Autodesk Fusion 360 part; units mm, degrees
sketch "Sketch1" plane through (0, 0, 0) normal (0, 0, 1) x (1, 0, 0)
  line L0 (-27.1259, 29.8327) -> (51.8741, 29.8327)
  line L1 (51.8741, 29.8327) -> (51.8741, -62.1673)
  line L2 (51.8741, -62.1673) -> (-27.1259, -62.1673)
  line L3 (-27.1259, -62.1673) -> (-27.1259, 29.8327)
  line L4 (62.3741, -72.1673) -> (-36.6259, -72.1673)
  line L5 (-36.6259, -72.1673) -> (-36.6259, 39.8327)
  line L6 (-36.6259, 39.8327) -> (62.3741, 39.8327)
  line L7 (62.3741, 39.8327) -> (62.3741, -72.1673)
  line L8 (62.3741, -72.1673) -> (-36.6259, 39.8327) construction
  line L9 (-36.6259, -72.1673) -> (62.3741, 39.8327) construction
  circle A0 centre (-31.6259, -67.1673) radius 1.7
  circle A1 centre (-31.6259, 34.8327) radius 1.7
  circle A2 centre (57.3741, 34.8327) radius 1.7
  circle A3 centre (57.3741, -67.1673) radius 1.7
  circle A4 centre (-31.6259, 34.8327) radius 3
  circle A5 centre (57.3741, 34.8327) radius 3
  circle A6 centre (57.3741, -67.1673) radius 3
  circle A7 centre (-31.6259, -67.1673) radius 3
  point P0 (12.8741, -16.1673)
  dimension "d1" = 79
  dimension "d3" = 99
  dimension "d4" = 112
  dimension "d13" = 3.4
  dimension "d14" = 5
  dimension "d15" = 5
  dimension "d16" = 9.5
  dimension "d17" = 6
  dimension "d18" = 6
  dimension "d19" = 6
  dimension "d20" = 6
extrude "Extrude1" add sketch "Sketch1" along normal blind 9.9 from surface at 3.1 contours A4 | A5 | A6 | A7 makes body 1 at (-34.6222, 34.6832, 9.7) makes body 2 at (-34.3904, -68.3326, 9.7) makes body 3 at (54.3778, 34.6832, 9.7) makes body 4 at (54.8142, -68.7316, 9.7)
extrude "Extrude2" add sketch "Sketch1" along normal blind 13 contours L4 L5 L6 L7 bodies 1 2 3 4
extrude "Extrude3" add sketch "Sketch1" along normal blind 3 contours L0 L1 L2 L3 bodies 1
sketch "Sketch2" plane through (0, 0, 13) normal (0, 0, 1) x (-1, 0, 0)
  circle A0 centre (31.6259, -34.8327) radius 1.7
  circle A1 centre (-57.3741, 67.1673) radius 1.7
  line L0 (-51.8741, 62.1673) -> (27.1259, 62.1673)
  line L1 (27.1259, 62.1673) -> (27.1259, -29.8327)
  line L2 (27.1259, -29.8327) -> (-51.8741, -29.8327)
  line L3 (-51.8741, -29.8327) -> (-51.8741, 62.1673)
  line L4 (-62.3741, -39.8327) -> (36.6259, -39.8327)
  line L5 (36.6259, -39.8327) -> (36.6259, 72.1673)
  line L6 (36.6259, 72.1673) -> (-62.3741, 72.1673)
  line L7 (-62.3741, 72.1673) -> (-62.3741, -39.8327)
  circle A2 centre (31.6259, 67.1673) radius 1.7
  circle A3 centre (-57.3741, -34.8327) radius 1.7
  line L8 (-3.6241, 62.1673) -> (-22.1241, 62.1673)
  line L9 (-22.1241, 62.1673) -> (-22.1241, 72.1673)
  line L10 (-22.1241, 72.1673) -> (-3.6241, 72.1673)
  line L11 (-3.6241, 72.1673) -> (-3.6241, 62.1673)
  line L12 (-3.6241, 62.1673) -> (-22.1241, 72.1673) construction
  line L13 (-22.1241, 62.1673) -> (-3.6241, 72.1673) construction
  point P0 (-12.8741, 67.1673)
  dimension "d28" = 18.5
extrude "Extrude4" cut sketch "Sketch2" against normal blind 7.5 contours L0 L6 L8 L9 L10 L11 bodies 1
fillet "Fillet1" radius 5 1 edges at (-36.6259, 39.8327, 6.5) on bodies 1
fillet "Fillet2" radius 5 3 edges at (62.3741, 39.8327, 6.5) (62.3741, -72.1673, 6.5) (-36.6259, -72.1673, 6.5) on bodies 1
Model file for the job. Use its own axes, mm. A direction names the side the tool comes from. Round coordinates to 2 decimals unless told otherwise and drop trailing zeros. Loops run counter-clockwise (first coordinate to the right, second up) from the corner with the lowest first, then second, coordinate; pieces in that order, holes last. Notation, with made-up numbers: M 54,-12.5 L 111,-12.5 A20 cw 111,-8.5 Z; hole C 39.5,44 d4. An arc over 180 degrees is marked long. Put each result on its own line as item: value. Start each with the question number.
Item 1: 3-axis set-ups, long thin cutter, end or side, ignore diameter. For faces 1 (the face through (12, 29.833, 8)), 2 (the face through (58.7, 33.5, 3.1)), 3 (the face through (-36.626, -17, 6)), 4 (the face through (3.624, -67, 9)): which of +Z, -Z, +X, -X, +Y, -Y reach the whole face in a straight line?
Item 2: Cut at A-A (z = 8.25). List the corners of the cut face in (x, y), then the cut area to 3 significant figures.
Item 3: Drop a flat-ended pin along its axis: P1, Ø3, axis at x = -30.5, y = 35.5, coming from the -Z side. Give the stop position or say it passes through.
Item 4: Cut at C-C (y = -60.5). List the corners of the cut face in (x, z), then the cut area to 3 significant figures.
Item 5: Drill centre lines: line 1 along X through (y, z) = (16, 4.5); line 2 along Y through (x, z) = (44, 5.5); line 3 along Y through (x, z) = (-30.5, 11.5). Where is each one in solid material? Low to high.
Item 6: Cut at B-B (x = 10.5). List the corners of the cut face in (y, z), then the cut area to 3 significant figures.
Item 7: Mould opens along Y. For faces 5 (the face through (22.124, -67, 9)), 6 (the face through (60.95, 38.33, 6.59)), 7 (the face through (-34.623, 34.701, 1.528)), 8 (the face through (13, -62.167, 5)) say: released by +Y, released by -Y, zero draft, split by the parting line, or undercut.
Answer block:
1. face 1: +Z
1. face 2: -Z
1. face 3: +Z, -Z, -X, +Y, -Y
1. face 4: +Z, -Y
2. outline: M -36.63,-67.17 A5 ccw -31.63,-72.17 L 3.62,-72.17 L 3.62,-62.17 L -27.13,-62.17 L -27.13,29.83 L 51.87,29.83 L 51.87,-62.17 L 22.12,-62.17 L 22.12,-72.17 L 57.37,-72.17 A5 ccw 62.37,-67.17 L 62.37,34.83 A5 ccw 57.37,39.83 L -31.63,39.83 A5 ccw -36.63,34.83 Z; hole C -31.63,-67.17 d3.4; hole C -31.63,34.83 d3.4; hole C 57.37,-67.17 d3.4; hole C 57.37,34.83 d3.4
2. area: 3,580 mm2
3. P1: z = 3.1
4. outline: M -36.63,0 L 62.37,0 L 62.37,13 L 51.87,13 L 51.87,3 L -27.13,3 L -27.13,13 L -36.63,13 Z
4. area: 497 mm2
5. line 1: -36.63 to -27.13, 51.87 to 62.37
5. line 2: -72.17 to -62.17, 29.83 to 39.83
5. line 3: -72.17 to -68.44, -65.89 to 33.56, 36.11 to 39.83
6. outline: M -72.17,0 L 39.83,0 L 39.83,13 L 29.83,13 L 29.83,3 L -62.17,3 L -62.17,5.5 L -72.17,5.5 Z
6. area: 461 mm2
7. face 5: zero draft
7. face 6: released by +Y
7. face 7: undercut
7. face 8: undercut
